Can you work these out from the drawing? Everything is in mm from the part's minimum corner. Coordinates: 2 decimals unless noted, no trailing zeros. Order: outer loops, then holes, each group sorted by start corner. A loop starts at its lowest first (then second) coordinate and runs counter-clockwise, first axis right, second up. Notation, with made-up numbers: (61, -18) - (109, -18) arc R26 cw to (109, 8) - close; hole circle Ø7 at (-13.5, -10). An arc over 180 degrees is marked (long way). Use one line per item in the form item = value. Start each with the question number.
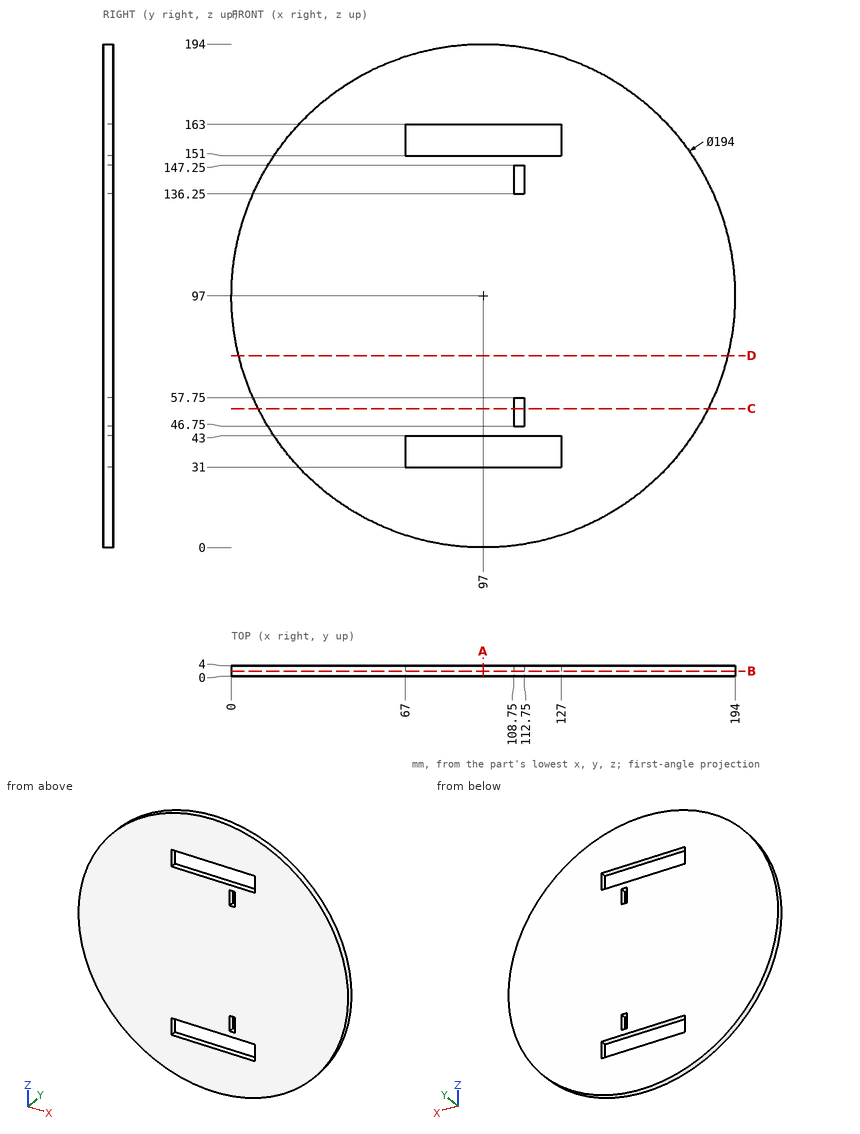
1) Suppose I cut it at A-A, the plane x = 97. List the corners of the cut face in (y, z) for me.
2) Suppose I cut it at D-D, the plane z = 74. List the corners of the cut face in (x, y) for me, then the cut area to 3 significant figures.
3) Suppose I cut it at C-C, the plane z = 53.5. List the corners of the cut face in (x, y) for me.
4) Suppose I cut it at B-B, the plane y = 1.9. List the corners of the cut face in (x, z) for me.
5) For pin 1 (2 mm diameter, centred on y = 3, z = 157.5, fed in from +X); pin 2 (2 mm diameter, centred on y = 2.5, z = 50, fed in from -X); pin 3 (1 mm diameter, centred on y = 1.5, z = 23.5, fed in from +X); pin 4 (1 mm diameter, centred on x = 84.5, z = 29, fed in from -Y), each with a flat end and sliding along its axis, tell me the tip position at first contact or that it passes through.
6) I need wall thicknesses on probe 1 along Z at (x, y) = (110, 3.2); probe 2 along Z at (x, y) = (111.5, 0.95); probe 3 along X at (y, z) = (1.5, 141). Which ranges of each line are inside material? Lowest first, please. Write a range as [from, to].
From the geometry:
q1.outline = (0, 0) - (4, 0) - (4, 31) - (0, 31) - close; (0, 43) - (4, 43) - (4, 151) - (0, 151) - close; (0, 163) - (4, 163) - (4, 194) - (0, 194) - close
q2.outline = (2.77, 0) - (191.23, 0) - (191.23, 4) - (2.77, 4) - close
q2.area = 754 mm2
q3.outline = (10.3, 0) - (108.75, 0) - (108.75, 4) - (10.3, 4) - close; (112.75, 0) - (183.7, 0) - (183.7, 4) - (112.75, 4) - close
q4.outline = circle Ø194 at (97, 97); hole (67, 31) - (127, 31) - (127, 43) - (67, 43) - close; hole (67, 151) - (127, 151) - (127, 163) - (67, 163) - close; hole (108.75, 46.75) - (112.75, 46.75) - (112.75, 57.75) - (108.75, 57.75) - close; hole (108.75, 136.25) - (112.75, 136.25) - (112.75, 147.25) - (108.75, 147.25) - close
q5.pin_1 = 173.61
q5.pin_2 = 11.6
q5.pin_3 = 160.87
q5.pin_4 = 0
q6.probe_1 = [0.88, 31], [43, 46.75], [57.75, 136.25], [147.25, 151], [163, 193.12]
q6.probe_2 = [1.09, 31], [43, 46.75], [57.75, 136.25], [147.25, 151], [163, 192.91]
q6.probe_3 = [10.55, 108.75], [112.75, 183.45]
